Model file for the job. Use its own axes, mm. A direction names the side the tool comes from. Coordinates: 2 decimals unless noted, no trailing zeros. Order: outer loops, then holes, each group sorted by start corner. A loop starts at its lowest first (then second) coordinate and runs counter-clockwise, first axis right, second up. Notation, with made-up numbers: (-25, 80.25) -> (27, 80.25) arc R17 cw to (27, 87.25) -> close; hole circle Ø5 at (-9, -32.75). An arc over 180 degrees is marked (long way). Write item = value, one per line. Start each with the question number.
Q1. Wall check: line 1 (Z direction, x = -6, y = -3); line 2 (Z direction, x = -11.5, y = -4.5); line 3 (Y direction, x = -16, z = 1.25). Give the ranges that are in metal, low to high. Write a range as from..to.
Q2. Cut at D-D, the plane x = -16. List the corners of the cut face in (y, z), plus the area to 3 significant figures.
Q3. Flat gauge pins, fed straight in: pin 1 (8 mm diameter, centred on y = 6, z = 1, fed in from -X); pin 2 (3 mm diameter, centred on y = 13, z = 3, fed in from +X); pin 3 (6 mm diameter, centred on x = -11, z = 6, fed in from +Y). Where does each tip first touch, or does it go through?
Q4. Cut at C-C, the plane y = 19.5. List the corners of the cut face in (x, z), plus the area to 3 significant figures.
Q5. 3-axis set-ups, long thin cutter, end or side, ignore diameter. For faces 4 (the face through (3.695, -1.163, -4.383)), 5 (the face through (17.99, -7.25, 1.25)), 6 (the face through (-10, -5, 2.54)): which of +Z, -Z, +X, -X, +Y, -Y reach the whole face in a straight line?
Q6. Mould opens along Y. For faces 1 (the face through (0, 0, -8.89)), 2 (the face through (-12.292, -10.406, 1.252)), 3 (the face through (10.48, 3.3, 10.8)) say: +Y half, -Y half, draft (parallel to the pull), parting line (faces both ways), or undercut.
Q7. Cut at A-A, the plane x = 0. List the corners of the cut face in (y, z).
Q8. Cut at B-B, the plane y = 0. List the corners of the cut face in (x, z), plus the area to 3 significant figures.
from build123d import *

# Parameters (mm, degrees)
SKETCH1_R           = 21.9075
SKETCH1_R_2         = 2.610660844
BOSS_EXTRUDE1_DEPTH = 2.54
SKETCH2_R           = 3.8735
BOSS_EXTRUDE2_DEPTH = 8.89
SKETCH3_R           = 10.9855
BOSS_EXTRUDE4_DEPTH = 16.764


with BuildPart() as part:
    # Sketch1 → Boss-Extrude1 (new body)
    with BuildSketch(Plane.XY):
        Circle(SKETCH1_R)
        with Locations((-0.793799024, 17.4371)):
            Circle(SKETCH1_R_2, mode=Mode.SUBTRACT)
        with Locations((15.49787108, -8.03109988)):
            Circle(SKETCH1_R_2, mode=Mode.SUBTRACT)
        with Locations((-14.704072056, -9.40600012)):
            Circle(SKETCH1_R_2, mode=Mode.SUBTRACT)
    extrude(amount=BOSS_EXTRUDE1_DEPTH)

    # Sketch2 → Boss-Extrude2 (add)
    with BuildSketch(Plane(origin=(0, 0, 0), x_dir=(-1, 0, 0), z_dir=(0, 0, -1))):
        with Locations(Location((0, 0, 0), (0, 0, 180))):
            Circle(SKETCH2_R)
    extrude(amount=BOSS_EXTRUDE2_DEPTH)

    # Sketch3 → Boss-Extrude4 (add)
    with BuildSketch(Plane.XY.offset(2.54)):
        Circle(SKETCH3_R)
    extrude(amount=BOSS_EXTRUDE4_DEPTH)


solid = part.part
Here are the results:
q1.line_1 = 0..19.3
q1.line_2 = 0..2.54
q1.line_3 = -14.96..-11.67, -7.14..14.96
q2.outline = (-14.96, 0) -> (-11.67, 0) -> (-11.67, 2.54) -> (-14.96, 2.54) -> close; (-7.14, 0) -> (14.96, 0) -> (14.96, 2.54) -> (-7.14, 2.54) -> close
q2.area = 64.5 mm²
q3.pin_1 = -21.82
q3.pin_2 = 18.6
q3.pin_3 = 7.53
q4.outline = (-9.98, 0) -> (-2.39, 0) -> (-2.39, 2.54) -> (-9.98, 2.54) -> close; (0.81, 0) -> (9.98, 0) -> (9.98, 2.54) -> (0.81, 2.54) -> close
q4.area = 42.6 mm²
q5.face_4 = -Z
q5.face_5 = +Z, -Z
q5.face_6 = +Z
q6.face_1 = draft
q6.face_2 = undercut
q6.face_3 = parting line
q7.outline = (-21.91, 0) -> (-3.87, 0) -> (-3.87, -8.89) -> (3.87, -8.89) -> (3.87, 0) -> (14.95, 0) -> (14.95, 2.54) -> (10.99, 2.54) -> (10.99, 19.3) -> (-10.99, 19.3) -> (-10.99, 2.54) -> (-21.91, 2.54) -> close; (19.92, 0) -> (21.91, 0) -> (21.91, 2.54) -> (19.92, 2.54) -> close
q8.outline = (-21.91, 0) -> (-3.87, 0) -> (-3.87, -8.89) -> (3.87, -8.89) -> (3.87, 0) -> (21.91, 0) -> (21.91, 2.54) -> (10.99, 2.54) -> (10.99, 19.3) -> (-10.99, 19.3) -> (-10.99, 2.54) -> (-21.91, 2.54) -> close
q8.area = 548 mm²
